For this review, take the finished solid that the model builds, in its own axes (mm). Face numbers are marked on the shaded views. Give positions to 0.01 mm unless a question says otherwise; leave off trailing zeros. Loops run counter-clockwise (first coordinate to the right, second up) from the corner with the lowest first, then second, coordinate; pieces in that order, holes last. Notation, with made-up numbers: (79.25, 51.25) - (108.25, 51.25) arc R14 cw to (108.25, 56.25) - close; hole circle Ø3 at (49, 41). An arc over 180 degrees is marked (long way). Answer as CSV lines item,"result".
from build123d import *

# Parameters (mm, degrees)
SKETCH1_R           = 6
BOSS_EXTRUDE1_DEPTH = 35
CUT_EXTRUDE5_START  = -4.5
CUT_EXTRUDE5_DEPTH  = 4.5
SKETCH6_R           = 6.880488524
SKETCH6_R_2         = 4.4323
CUT_EXTRUDE6_DEPTH  = 2.032
SKETCH7_R           = 3.4925
CUT_EXTRUDE7_DEPTH  = 7.112


# Read off the part's stored shape, not the designer's step: Cut-Extrude5
with BuildPart() as part:
    # Sketch1 → Boss-Extrude1 (new body)
    with BuildSketch(Plane.XY):
        Circle(SKETCH1_R)
    extrude(amount=-BOSS_EXTRUDE1_DEPTH)

    # Cut-Extrude5 outline → Cut-Extrude5 (cut)
    with BuildSketch(Plane.XY.offset(CUT_EXTRUDE5_START)):
        with BuildLine():
            ThreePointArc((5.992919203, -0.291409379), (6, 0), (5.992919203, 0.291409379))
            Line((5.992919203, 0.291409379), (5.5808372, 0))
            Line((5.5808372, 0), (5.992919203, -0.291409379))
        make_face()
        with BuildLine():
            Line((5.496051743, 0.96910221), (5.952476002, 0.753677283))
            ThreePointArc((5.952476002, 0.753677283), (5.908846518, 1.041889066), (5.851270587, 1.327641714))
            Line((5.851270587, 1.327641714), (5.496051743, 0.96910221))
        make_face()
        with BuildLine():
            ThreePointArc((5.851270587, -1.327641714), (5.908846518, -1.041889066), (5.952476002, -0.753677283))
            Line((5.952476002, -0.753677283), (5.496051743, -0.96910221))
            Line((5.496051743, -0.96910221), (5.851270587, -1.327641714))
        make_face()
        with BuildLine():
            Line((5.244271535, 1.908758739), (5.73116983, 1.775863842))
            ThreePointArc((5.73116983, 1.775863842), (5.638155725, 2.05212086), (5.531834074, 2.323534328))
            Line((5.531834074, 2.323534328), (5.244271535, 1.908758739))
        make_face()
        with BuildLine():
            ThreePointArc((5.531834074, -2.323534328), (5.638155725, -2.05212086), (5.73116983, -1.775863842))
            Line((5.73116983, -1.775863842), (5.244271535, -1.908758739))
            Line((5.244271535, -1.908758739), (5.531834074, -2.323534328))
        make_face()
        with BuildLine():
            Line((4.83314679, 2.7904186), (5.335724962, 2.744091676))
            ThreePointArc((5.335724962, 2.744091676), (5.196152423, 3), (5.044315583, 3.248827527))
            Line((5.044315583, 3.248827527), (4.83314679, 2.7904186))
        make_face()
        with BuildLine():
            ThreePointArc((5.044315583, -3.248827527), (5.196152423, -3), (5.335724962, -2.744091676))
            Line((5.335724962, -2.744091676), (4.83314679, -2.7904186))
            Line((4.83314679, -2.7904186), (5.044315583, -3.248827527))
        make_face()
        with BuildLine():
            Line((4.275169325, 3.587293004), (4.778156792, 3.628941674))
            ThreePointArc((4.778156792, 3.628941674), (4.596266659, 3.856725658), (4.403528115, 4.075406745))
            Line((4.403528115, 4.075406745), (4.275169325, 3.587293004))
        make_face()
        with BuildLine():
            ThreePointArc((4.403528115, -4.075406745), (4.596266659, -3.856725658), (4.778156792, -3.628941674))
            Line((4.778156792, -3.628941674), (4.275169325, -3.587293004))
            Line((4.275169325, -3.587293004), (4.403528115, -4.075406745))
        make_face()
        with BuildLine():
            Line((3.587293004, 4.275169325), (4.075406745, 4.403528115))
            ThreePointArc((4.075406745, 4.403528115), (3.856725658, 4.596266659), (3.628941674, 4.778156792))
            Line((3.628941674, 4.778156792), (3.587293004, 4.275169325))
        make_face()
        with BuildLine():
            ThreePointArc((3.628941674, -4.778156792), (3.856725658, -4.596266659), (4.075406745, -4.403528115))
            Line((4.075406745, -4.403528115), (3.587293004, -4.275169325))
            Line((3.587293004, -4.275169325), (3.628941674, -4.778156792))
        make_face()
        with BuildLine():
            Line((2.7904186, 4.83314679), (3.248827527, 5.044315583))
            ThreePointArc((3.248827527, 5.044315583), (3, 5.196152423), (2.744091676, 5.335724962))
            Line((2.744091676, 5.335724962), (2.7904186, 4.83314679))
        make_face()
        with BuildLine():
            ThreePointArc((2.744091676, -5.335724962), (3, -5.196152423), (3.248827527, -5.044315583))
            Line((3.248827527, -5.044315583), (2.7904186, -4.83314679))
            Line((2.7904186, -4.83314679), (2.744091676, -5.335724962))
        make_face()
        with BuildLine():
            Line((1.908758739, 5.244271535), (2.323534328, 5.531834074))
            ThreePointArc((2.323534328, 5.531834074), (2.05212086, 5.638155725), (1.775863842, 5.73116983))
            Line((1.775863842, 5.73116983), (1.908758739, 5.244271535))
        make_face()
        with BuildLine():
            ThreePointArc((1.775863842, -5.73116983), (2.05212086, -5.638155725), (2.323534328, -5.531834074))
            Line((2.323534328, -5.531834074), (1.908758739, -5.244271535))
            Line((1.908758739, -5.244271535), (1.775863842, -5.73116983))
        make_face()
        with BuildLine():
            Line((0.96910221, 5.496051743), (1.327641714, 5.851270587))
            ThreePointArc((1.327641714, 5.851270587), (1.041889066, 5.908846518), (0.753677283, 5.952476002))
            Line((0.753677283, 5.952476002), (0.96910221, 5.496051743))
        make_face()
        with BuildLine():
            ThreePointArc((0.753677283, -5.952476002), (1.041889066, -5.908846518), (1.327641714, -5.851270587))
            Line((1.327641714, -5.851270587), (0.96910221, -5.496051743))
            Line((0.96910221, -5.496051743), (0.753677283, -5.952476002))
        make_face()
        with BuildLine():
            Line((0, 5.5808372), (0.291409379, 5.992919203))
            ThreePointArc((0.291409379, 5.992919203), (0, 6), (-0.291409379, 5.992919203))
            Line((-0.291409379, 5.992919203), (0, 5.5808372))
        make_face()
        with BuildLine():
            ThreePointArc((-0.291409379, -5.992919203), (0, -6), (0.291409379, -5.992919203))
            Line((0.291409379, -5.992919203), (0, -5.5808372))
            Line((0, -5.5808372), (-0.291409379, -5.992919203))
        make_face()
        with BuildLine():
            Line((-0.96910221, 5.496051743), (-0.753677283, 5.952476002))
            ThreePointArc((-0.753677283, 5.952476002), (-1.041889066, 5.908846518), (-1.327641714, 5.851270587))
            Line((-1.327641714, 5.851270587), (-0.96910221, 5.496051743))
        make_face()
        with BuildLine():
            ThreePointArc((-1.327641714, -5.851270587), (-1.041889066, -5.908846518), (-0.753677283, -5.952476002))
            Line((-0.753677283, -5.952476002), (-0.96910221, -5.496051743))
            Line((-0.96910221, -5.496051743), (-1.327641714, -5.851270587))
        make_face()
        with BuildLine():
            Line((-1.908758739, 5.244271535), (-1.775863842, 5.73116983))
            ThreePointArc((-1.775863842, 5.73116983), (-2.05212086, 5.638155725), (-2.323534328, 5.531834074))
            Line((-2.323534328, 5.531834074), (-1.908758739, 5.244271535))
        make_face()
        with BuildLine():
            ThreePointArc((-2.323534328, -5.531834074), (-2.05212086, -5.638155725), (-1.775863842, -5.73116983))
            Line((-1.775863842, -5.73116983), (-1.908758739, -5.244271535))
            Line((-1.908758739, -5.244271535), (-2.323534328, -5.531834074))
        make_face()
        with BuildLine():
            Line((-2.7904186, 4.83314679), (-2.744091676, 5.335724962))
            ThreePointArc((-2.744091676, 5.335724962), (-3, 5.196152423), (-3.248827527, 5.044315583))
            Line((-3.248827527, 5.044315583), (-2.7904186, 4.83314679))
        make_face()
        with BuildLine():
            ThreePointArc((-3.248827527, -5.044315583), (-3, -5.196152423), (-2.744091676, -5.335724962))
            Line((-2.744091676, -5.335724962), (-2.7904186, -4.83314679))
            Line((-2.7904186, -4.83314679), (-3.248827527, -5.044315583))
        make_face()
        with BuildLine():
            Line((-3.587293004, 4.275169325), (-3.628941674, 4.778156792))
            ThreePointArc((-3.628941674, 4.778156792), (-3.856725658, 4.596266659), (-4.075406745, 4.403528115))
            Line((-4.075406745, 4.403528115), (-3.587293004, 4.275169325))
        make_face()
        with BuildLine():
            ThreePointArc((-4.075406745, -4.403528115), (-3.856725658, -4.596266659), (-3.628941674, -4.778156792))
            Line((-3.628941674, -4.778156792), (-3.587293004, -4.275169325))
            Line((-3.587293004, -4.275169325), (-4.075406745, -4.403528115))
        make_face()
        with BuildLine():
            Line((-4.275169325, 3.587293004), (-4.403528115, 4.075406745))
            ThreePointArc((-4.403528115, 4.075406745), (-4.596266659, 3.856725658), (-4.778156792, 3.628941674))
            Line((-4.778156792, 3.628941674), (-4.275169325, 3.587293004))
        make_face()
        with BuildLine():
            ThreePointArc((-4.778156792, -3.628941674), (-4.596266659, -3.856725658), (-4.403528115, -4.075406745))
            Line((-4.403528115, -4.075406745), (-4.275169325, -3.587293004))
            Line((-4.275169325, -3.587293004), (-4.778156792, -3.628941674))
        make_face()
        with BuildLine():
            Line((-4.83314679, 2.7904186), (-5.044315583, 3.248827527))
            ThreePointArc((-5.044315583, 3.248827527), (-5.196152423, 3), (-5.335724962, 2.744091676))
            Line((-5.335724962, 2.744091676), (-4.83314679, 2.7904186))
        make_face()
        with BuildLine():
            ThreePointArc((-5.335724962, -2.744091676), (-5.196152423, -3), (-5.044315583, -3.248827527))
            Line((-5.044315583, -3.248827527), (-4.83314679, -2.7904186))
            Line((-4.83314679, -2.7904186), (-5.335724962, -2.744091676))
        make_face()
        with BuildLine():
            Line((-5.244271535, 1.908758739), (-5.531834074, 2.323534328))
            ThreePointArc((-5.531834074, 2.323534328), (-5.638155725, 2.05212086), (-5.73116983, 1.775863842))
            Line((-5.73116983, 1.775863842), (-5.244271535, 1.908758739))
        make_face()
        with BuildLine():
            ThreePointArc((-5.73116983, -1.775863842), (-5.638155725, -2.05212086), (-5.531834074, -2.323534328))
            Line((-5.531834074, -2.323534328), (-5.244271535, -1.908758739))
            Line((-5.244271535, -1.908758739), (-5.73116983, -1.775863842))
        make_face()
        with BuildLine():
            Line((-5.496051743, 0.96910221), (-5.851270587, 1.327641714))
            ThreePointArc((-5.851270587, 1.327641714), (-5.908846518, 1.041889066), (-5.952476002, 0.753677283))
            Line((-5.952476002, 0.753677283), (-5.496051743, 0.96910221))
        make_face()
        with BuildLine():
            ThreePointArc((-5.952476002, -0.753677283), (-5.908846518, -1.041889066), (-5.851270587, -1.327641714))
            Line((-5.851270587, -1.327641714), (-5.496051743, -0.96910221))
            Line((-5.496051743, -0.96910221), (-5.952476002, -0.753677283))
        make_face()
        with BuildLine():
            Line((-5.5808372, 0), (-5.992919203, 0.291409379))
            ThreePointArc((-5.992919203, 0.291409379), (-6, 0), (-5.992919203, -0.291409379))
            Line((-5.992919203, -0.291409379), (-5.5808372, 0))
        make_face()
    extrude(amount=CUT_EXTRUDE5_DEPTH, mode=Mode.SUBTRACT)

    # Sketch6 → Cut-Extrude6 (cut)
    with BuildSketch(Plane.XY.offset(-4.5)):
        Circle(SKETCH6_R)
        Circle(SKETCH6_R_2, mode=Mode.SUBTRACT)
    extrude(amount=-CUT_EXTRUDE6_DEPTH, mode=Mode.SUBTRACT)

    # Sketch7 → Cut-Extrude7 (cut)
    with BuildSketch(Plane.XY):
        Circle(SKETCH7_R)
    extrude(amount=-CUT_EXTRUDE7_DEPTH, mode=Mode.SUBTRACT)


solid = part.part
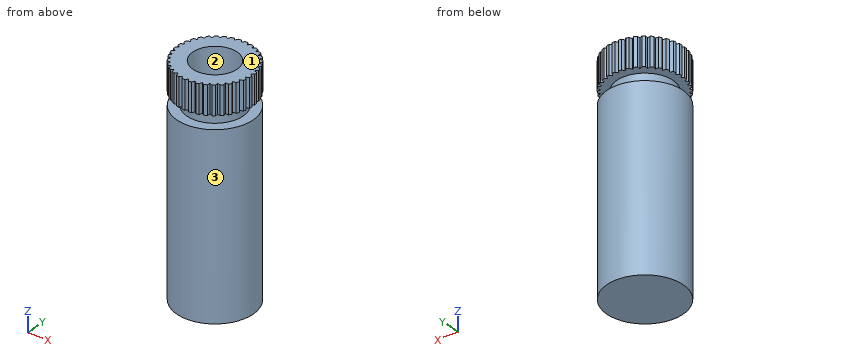
1) Insertion check: P1, Ø2, axis at y = 2, z = -22.5, coming from the -X side; P2, Ø2, axis at y = 4.5, z = -31, coming from the +X side; P3, Ø5, axis at y = -2, z = -4.5, coming from the -X side. Each pin has a flat end and moves straight along its axis. Give the tip position at first contact, or say it passes through.
From the geometry:
P1,"stops at x = -5.92"
P2,"stops at x = 4.87"
P3,"stops at x = -5.99"
2) Consider section B-B on z = -24. Write out the cut boundary in (x, y), and give its area (3 significant figures).
From the geometry:
outline,"circle Ø12 at (0, 0)"
area,"113 mm^2"
3) Draft analysis for pull direction Y (two halves, no side actions). For the marked faces 1, 2 and 3, state which applies: pulls with the +Y half, pulls with the -Y half, needs draft (parallel to the pull), parting line crosses it, or undercut.
From the geometry:
face 1,"needs draft"
face 2,"undercut"
face 3,"parting line crosses it"
4) Wall thickness on line 1 (Y direction, x = 0, z = -4.75); line 2 (Z direction, x = 0.5, y = 5.25); line 3 (Z direction, x = -3, y = -5): over which ranges is each line inside the solid? List them lowest first. Write a range as from..to.
From the geometry:
line 1,"y = -4.43..-3.49, 3.49..4.43"
line 2,"z = -35..-6.53, -4.5..0"
line 3,"z = -35..-6.53"
5) Consider section A-A on z = -5. Write out the cut boundary in (x, y) (1 decimal).
From the geometry:
outline,"circle Ø8.9 at (0, 0); hole circle Ø7 at (0, 0)"
